Geometry: final body of the model. Coordinates: model frame, mm. Coordinates: 2 decimals unless noted, no trailing zeros. Write each loop counter-clockwise with the first axis right and the second up, starting at its lowest first coordinate (ties: lowest second). Pieces come first, ordered by that corner, then holes.
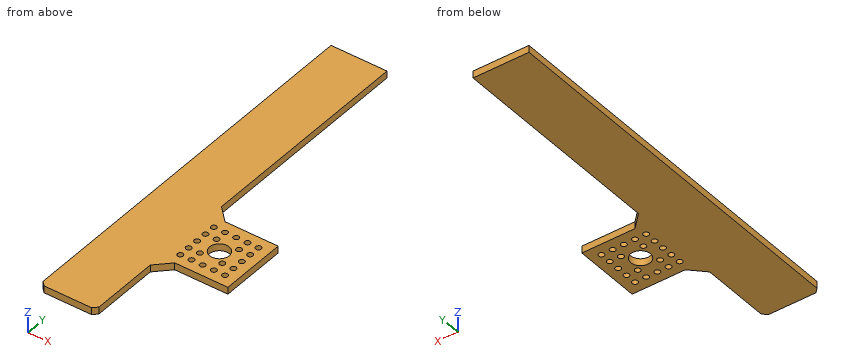
from build123d import *

# Parameters (mm, degrees)
SKETCH1_R           = 7
SKETCH1_R_2         = 2
BOSS_EXTRUDE1_DEPTH = 5
CHAMFER2_SIZE       = 3
CHAMFER3_SIZE       = 10


with BuildPart() as part:
    # Sketch1 → Boss-Extrude1 (new body)
    with BuildSketch(Plane.XY):
        Polygon((0, 0), (0, -278), (40, -278), (40, -216), (88, -216), (88, -168), (40, -168), (40, 0), align=None)
        with Locations((64, -192)):
            Circle(SKETCH1_R, mode=Mode.SUBTRACT)
        with Locations((48, -176)):
            Circle(SKETCH1_R_2, mode=Mode.SUBTRACT)
        with Locations((56, -176)):
            Circle(SKETCH1_R_2, mode=Mode.SUBTRACT)
        with Locations((64, -176)):
            Circle(SKETCH1_R_2, mode=Mode.SUBTRACT)
        with Locations((72, -176)):
            Circle(SKETCH1_R_2, mode=Mode.SUBTRACT)
        with Locations((80, -176)):
            Circle(SKETCH1_R_2, mode=Mode.SUBTRACT)
        with Locations((56, -184)):
            Circle(SKETCH1_R_2, mode=Mode.SUBTRACT)
        with Locations((72, -184)):
            Circle(SKETCH1_R_2, mode=Mode.SUBTRACT)
        with Locations((80, -184)):
            Circle(SKETCH1_R_2, mode=Mode.SUBTRACT)
        with Locations((80, -192)):
            Circle(SKETCH1_R_2, mode=Mode.SUBTRACT)
        with Locations((56, -200)):
            Circle(SKETCH1_R_2, mode=Mode.SUBTRACT)
        with Locations((72, -200)):
            Circle(SKETCH1_R_2, mode=Mode.SUBTRACT)
        with Locations((80, -200)):
            Circle(SKETCH1_R_2, mode=Mode.SUBTRACT)
        with Locations((56, -208)):
            Circle(SKETCH1_R_2, mode=Mode.SUBTRACT)
        with Locations((64, -208)):
            Circle(SKETCH1_R_2, mode=Mode.SUBTRACT)
        with Locations((72, -208)):
            Circle(SKETCH1_R_2, mode=Mode.SUBTRACT)
        with Locations((80, -208)):
            Circle(SKETCH1_R_2, mode=Mode.SUBTRACT)
        with Locations((48, -184)):
            Circle(SKETCH1_R_2, mode=Mode.SUBTRACT)
        with Locations((48, -192)):
            Circle(SKETCH1_R_2, mode=Mode.SUBTRACT)
        with Locations((48, -200)):
            Circle(SKETCH1_R_2, mode=Mode.SUBTRACT)
        with Locations((48, -208)):
            Circle(SKETCH1_R_2, mode=Mode.SUBTRACT)
    extrude(amount=BOSS_EXTRUDE1_DEPTH)

    # Chamfer2
    chamfer2_edges = [part.edges().sort_by_distance(p)[0] for p in [
        (40, -278, 2.5),
        (0, -278, 2.5),
    ]]
    chamfer(chamfer2_edges, length=CHAMFER2_SIZE)

    # Chamfer3
    chamfer3_edges = [part.edges().sort_by_distance(p)[0] for p in [
        (40, -168, 2.5),
        (40, -216, 2.5),
    ]]
    chamfer(chamfer3_edges, length=CHAMFER3_SIZE)


solid = part.part
Item 1: Section B-B, the plane y = -141. Output: boundary loops of the cut face in (x, z).
Derived:
outline: (0, 0) - (40, 0) - (40, 5) - (0, 5) - close
Item 2: Section A-A, the plane z = 1.45. State how many separate pieces and enclosed holes the cut face has, plus the area to 3 significant figures.
Derived:
separate pieces: 1
enclosed holes: 21
area: 13,100 mm2
Item 3: Material intervals for probe 1 along X at (y, z) = (-200, 1.7); probe 2 along X at (y, z) = (-176, 1.9); probe 3 along Y at (x, z) = (56, 2.2), sorted ascending.
Derived:
probe 1: x = 0 to 46, 50 to 54, 58 to 70, 74 to 78, 82 to 88
probe 2: x = 0 to 46, 50 to 54, 58 to 62, 66 to 70, 74 to 78, 82 to 88
probe 3: y = -216 to -210, -206 to -202, -198 to -186, -182 to -178, -174 to -168
Item 4: Pin query (flat end, axial travel): pin 1 (3 mm diameter, centred on x = 48, y = -176, fed in from -Z); pin 2 (2.5 mm diameter, centred on x = 63.5, z = 2, fed in from -Y); pin 3 (2 mm diameter, centred on x = 76, z = 4.5, fed in from +Y). Return the tip coordinate at first contact, or that it passes through.
Derived:
pin 1: passes through
pin 2: stops at y = -216
pin 3: stops at y = -168
